CAD build for the part. Positions are in the model's coordinates, mm. Give positions to 0.01 mm unless a question says otherwise; leave off trailing zeros. Loops run counter-clockwise (first coordinate to the right, second up) from the corner with the lowest first, then second, coordinate; pieces in that order, holes last. Notation, with made-up numbers: M 76,65.25 L 118,65.25 A25 cw 118,84.25 Z; hole C 54,-30.75 d3. An arc over 180 degrees is marked long. One line per question, with ' | ' between items.
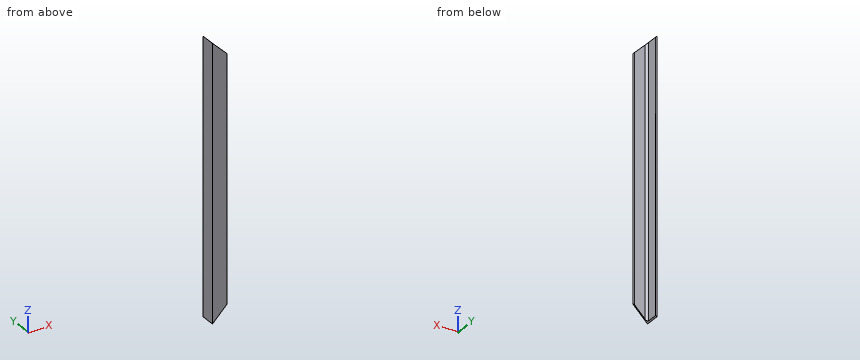
Autodesk Inventor part; units mm, degrees
ref_plane "Start plane" through (0, 0, -20) normal (0, 0, 1) x (1, 0, 0)
ref_plane "End plane" through (0, 0, 720) normal (0, 0, 1) x (1, 0, 0)
ref_plane "Work Plane11" through (-11.2, 8.8, -20) normal (0.7071, 0, -0.7071) x (-0.7071, 0, -0.7071)
ref_plane "Start plane" through (0, 0, -20) normal (0, 0, 1) x (1, 0, 0)
ref_plane "End plane" through (0, 0, 720) normal (0, 0, 1) x (1, 0, 0)
sketch "Sketch2" plane through (0, 0, 0) normal (0, 0, 1) x (1, 0, 0)
  line L0 (-8.2, -2.2) -> (-8.2, 25.8)
  line L1 (-11.2, 28.8) -> (-11.2, 28.8)
  line L2 (-11.2, -11.2) -> (-11.2, 28.8)
  line L3 (-11.2, -11.2) -> (28.8, -11.2)
  line L4 (28.8, -11.2) -> (28.8, -11.2)
  line L5 (-2.2, -8.2) -> (25.8, -8.2)
  arc A0 (-8.2, -2.2) -> (-2.2, -8.2) centre (-2.2, -2.2) ccw
  arc A1 (-8.2, 25.8) -> (-11.2, 28.8) centre (-11.2, 25.8) ccw
  arc A2 (28.8, -11.2) -> (25.8, -8.2) centre (25.8, -11.2) ccw
  line L6 (0, 37.5456) -> (0, -19.3243) construction
  line L7 (-19.3243, 0) -> (37.5456, 0) construction
  point P0 (-8.2, -8.2)
  point P1 (-8.2, 28.8)
  point P2 (28.8, -8.2)
  dimension "d4" = 40
  dimension "d6" = 40
  dimension "d8" = 3
  dimension "d10" = 3
  dimension "d17" = 6
  dimension "d18" = 3
  dimension "d19" = 11.2
  dimension "d20" = 11.2
extrude "Body" add sketch "Sketch2" along normal up to surface (740 mm away) from surface at -20
sketch "Sketch3" plane through (0, 0, 0) normal (0, 0, 1) x (1, 0, 0)
  line L0 (0, 0) -> (10, 0)
ref_plane "Work Plane10" through (0, 0, 0) normal (0, -1, 0) x (1, 0, 0)
sketch "Sketch4" plane through (0, 0, 0) normal (0, -1, 0) x (1, 0, 0)
  line L0 (-2, -20) -> (12, -20)
  line L1 (-2, 720) -> (12, 720)
  dimension "d24" = 740
ref_plane "Work Plane11" through (-11.2, 8.8, -20) normal (0.7071, 0, -0.7071) x (-0.7071, 0, -0.7071)
split "Split1" plane through (-11.2, 8.8, -20) removes the side toward (0.7071, 0, -0.7071)
ref_plane "Work Plane12" through (-11.2, 8.8, 720) normal (0.7071, 0, 0.7071) x (0.7071, 0, -0.7071)
split "Split2" plane through (-11.2, 8.8, 720) removes the side toward (0.7071, 0, 0.7071)
equation "\"d4\" = b"
equation "\"d6\" = b"
equation "\"d17\" = R"
equation "\"d18\" = R1"
equation "\"d19\" = ex"
equation "\"d20\" = d19"
equation "\"d11\" = G_L"
equation "\"b\" = 40"
equation "\"ParT\" = 3"
equation "\"R\" = 6"
equation "\"R1\" = 3"
equation "\"G_L\" = d24"
equation "\"ex\" = 11.2"
equation "\"G_OFFSET_START\" = 20"
equation "\"G_OFFSET_END\" = 20"
equation "\"d21\" = -G_OFFSET_START"
equation "\"d22\" = G_OFFSET_END + B_L"
equation "\"B_L\" = 700"
properties part number "ISO 657-1 - L40x40x3-740" material "Steel, Mild"
Item 1: Saw through at B-B on x = 18. Give the cut face in (y, z), and give its area (3 significant figures).
Conclusion:
outline: M -11.2,9.2 L -8.2,9.2 L -8.2,690.8 L -11.2,690.8 Z | area: 2,040 mm²
Item 2: Saw through at A-A on z = 553. Give the cut face in (x, y), and give its area (3 significant figures).
Conclusion:
outline: M -11.2,-11.2 L 28.8,-11.2 A3 ccw 25.8,-8.2 L -2.2,-8.2 A6 cw -8.2,-2.2 L -8.2,25.8 A3 ccw -11.2,28.8 Z | area: 235 mm²
Item 3: Drill centre lines: line 1 along Y through (x, z) = (2.5, 150); line 2 along Y through (x, z) = (-3, 155.5). Where is each one in solid material? Low to high. Write a range as [from, to].
Conclusion:
line 1: [-11.2, -8.2] | line 2: [-11.2, -8.15]
Item 4: Saw through at C-C on y = 8. Give the cut face in (x, z), and give its area (3 significant figures).
Conclusion:
outline: M -11.2,-20 L -8.2,-17 L -8.2,717 L -11.2,720 Z | area: 2,210 mm²
Item 5: Drop flat-ended pins along their axis: P1, Ø4, axis at x = 5.5, z = 372.5, coming from the +Y side; P2, Ø22.5, axis at y = 10, z = 363, coming from the +X side; P3, Ø3, axis at x = -5, y = 18.5, coming from the +Z side. Give the stop position or say it passes through.
Conclusion:
P1: y = -8.2 | P2: x = -8.2 | P3: through
